```python
from build123d import *

# Parameters (mm, degrees)
SKIZZE1_W                            = 12
SKIZZE1_H                            = 17
AUFSATZ_LINEAR_AUSTRAGEN1_DEPTH      = 2
SCHNITT_LINEAR_AUSTRAGEN1_DEPTH      = 21.90454496
SCHNITT_LINEAR_AUSTRAGEN1_DEPTH_BACK = 21.90454496
SKIZZE4_W                            = 3
SKIZZE4_H                            = 1
SCHNITT_LINEAR_AUSTRAGEN3_DEPTH      = 1
VERRUNDUNG1_R                        = 0.5
VERRUNDUNG2_R                        = 1.5
VERRUNDUNG3_R                        = 0.25


# Some blends are built 0.0001 mm under size
with BuildPart() as part:
    # Skizze1 → Aufsatz-Linear austragen1 (new body)
    with BuildSketch(Plane(origin=(0, 0, 0), x_dir=(1, 0, 0), z_dir=(0, 1, 0))):
        with Locations((6, 8.5)):
            Rectangle(SKIZZE1_W, SKIZZE1_H)
    extrude(amount=AUFSATZ_LINEAR_AUSTRAGEN1_DEPTH)

    # Skizze4 → Schnitt-Linear austragen1 (cut, two sides: drawn at the far end of the back side and taken through both)
    with BuildSketch(Plane(origin=(0, 2, 0), x_dir=(1, 0, 0), z_dir=(0, 1, 0)).offset(-SCHNITT_LINEAR_AUSTRAGEN1_DEPTH_BACK)):
        with Locations((8.5, 2.5)):
            Rectangle(SKIZZE4_W, SKIZZE4_H)
        with Locations((3.5, 14.5)):
            Rectangle(SKIZZE4_W, SKIZZE4_H)
    extrude(amount=SCHNITT_LINEAR_AUSTRAGEN1_DEPTH + SCHNITT_LINEAR_AUSTRAGEN1_DEPTH_BACK, mode=Mode.SUBTRACT)

    # Skizze3 → Schnitt-Linear austragen3 (cut)
    with BuildSketch(Plane(origin=(0, 2, 0), x_dir=(1, 0, 0), z_dir=(0, 1, 0))):
        Polygon((8, 4), (3, 4), (3, 9), (8, 9), (8, 12), (3, 12), (3, 14), (2, 14), (2, 11), (7, 11), (7, 10), (2, 10), (2, 3), (8, 3), align=None)
        Polygon((9, 5), (4, 5), (4, 8), (9, 8), (9, 13), (4, 13), (4, 14), (10, 14), (10, 7), (5, 7), (5, 6), (10, 6), (10, 3), (9, 3), align=None)
    extrude(amount=-SCHNITT_LINEAR_AUSTRAGEN3_DEPTH, mode=Mode.SUBTRACT)

    # Verrundung1
    verrundung1_edges = [part.edges().sort_by_distance(p)[0] for p in [
        (3, 1.5, -12),
        (3, 1.5, -9),
        (7, 1.5, -3),
        (5, 1.5, -14),
        (9, 1.5, -5),
        (9, 1.5, -8),
        (9, 1.5, -13),
        (5, 1.5, -7),
        (5, 1.5, -6),
        (3, 1.5, -4),
        (7, 1.5, -10),
        (7, 1.5, -11),
    ]]
    fillet(verrundung1_edges, radius=VERRUNDUNG1_R - 0.0001)  # a hair under: the kernel refuses the full size

    # Verrundung2
    # the kernel refuses this fillet: 1.5 mm, written as the material it adds along each edge
    with BuildSketch(Plane(origin=(4, 2, -8), x_dir=(0, 0, 1), z_dir=(0, -1, 0)), Plane(origin=(2, 2, -11), x_dir=(1, 0, 0), z_dir=(0, -1, 0)), Plane(origin=(2, 2, -3), x_dir=(1, 0, 0), z_dir=(0, -1, 0)), Plane(origin=(2, 2, -10), x_dir=(0, 0, 1), z_dir=(0, -1, 0)), Plane(origin=(4, 2, -5), x_dir=(1, 0, 0), z_dir=(0, -1, 0))) as verrundung2_piece_1:
        with BuildLine():
            CenterArc((VERRUNDUNG2_R, -VERRUNDUNG2_R), VERRUNDUNG2_R, 90, 90)
            Line((0, -VERRUNDUNG2_R), (-VERRUNDUNG2_R * 0.02, -VERRUNDUNG2_R))
            Line((-VERRUNDUNG2_R * 0.02, -VERRUNDUNG2_R), (-VERRUNDUNG2_R * 0.02, VERRUNDUNG2_R * 0.02))
            Line((-VERRUNDUNG2_R * 0.02, VERRUNDUNG2_R * 0.02), (VERRUNDUNG2_R, VERRUNDUNG2_R * 0.02))
            Line((VERRUNDUNG2_R, VERRUNDUNG2_R * 0.02), (VERRUNDUNG2_R, 0))
        make_face()
    extrude(amount=1)
    with BuildSketch(Plane(origin=(8, 2, -4), x_dir=(-1, 0, 0), z_dir=(0, -1, 0)), Plane(origin=(4, 2, -13), x_dir=(1, 0, 0), z_dir=(0, -1, 0))) as verrundung2_piece_2:
        with BuildLine():
            CenterArc((1.414213562, -1.5), VERRUNDUNG2_R, 90, 70.528779366)
            Line((0, -1), (-0.028284271, -0.99))
            ThreePointArc((-0.028284271, -0.99), (-0.03, -0.5), (-0.03, 0))
            Line((-0.03, 0), (0, 0.03))
            Line((0, 0.03), (1.414213562, 0.03))
            Line((1.414213562, 0.03), (1.414213562, 0))
        make_face()
    extrude(amount=1)
    with BuildSketch(Plane(origin=(10, 2, -14), x_dir=(0, 0, 1), z_dir=(0, -1, 0)), Plane(origin=(10, 2, -7), x_dir=(-1, 0, 0), z_dir=(0, -1, 0)), Plane(origin=(10, 2, -6), x_dir=(0, 0, 1), z_dir=(0, -1, 0)), Plane(origin=(8, 2, -12), x_dir=(0, 0, 1), z_dir=(0, -1, 0)), Plane(origin=(8, 2, -9), x_dir=(-1, 0, 0), z_dir=(0, -1, 0))) as verrundung2_piece_3:
        with BuildLine():
            CenterArc((VERRUNDUNG2_R, VERRUNDUNG2_R), VERRUNDUNG2_R, 180, 90)
            Line((0, VERRUNDUNG2_R), (-VERRUNDUNG2_R * 0.02, VERRUNDUNG2_R))
            Line((-VERRUNDUNG2_R * 0.02, VERRUNDUNG2_R), (-VERRUNDUNG2_R * 0.02, -VERRUNDUNG2_R * 0.02))
            Line((-VERRUNDUNG2_R * 0.02, -VERRUNDUNG2_R * 0.02), (VERRUNDUNG2_R, -VERRUNDUNG2_R * 0.02))
            Line((VERRUNDUNG2_R, -VERRUNDUNG2_R * 0.02), (VERRUNDUNG2_R, 0))
        make_face()
    extrude(amount=1)

    # Verrundung3
    verrundung3_edges = [part.edges().sort_by_distance(p)[0] for p in [
        (3, 1.5, -14),
        (2.5, 1, -14),
        (5, 1, -14.24995),
        (7, 1, -2.75005),
        (10, 1, -2),
        (7, 1, -2),
        (2, 1, -15),
        (5, 1, -15),
        (4, 1.5, -14),
        (9, 1.5, -3),
        (4.5, 1, -14),
        (9.5, 1, -3),
        (7.5, 1, -3),
        (8, 1.5, -3),
    ]]
    fillet(verrundung3_edges, radius=VERRUNDUNG3_R)


solid = part.part
```
Check sheet for the modelled part. Datum: model origin and axes. Units: mm. A direction names the side the tool comes from. Give positions to 0.01 mm unless a question says otherwise; leave off trailing zeros. Write each loop counter-clockwise with the first axis right and the second up, starting at its lowest first coordinate (ties: lowest second). Pieces come first, ordered by that corner, then holes.
Item 1: Scan lines: L1, parallel to X at y = 1.45, z = -8.5; L2, parallel to Z at x = 3.5, y = 1.7; L3, parallel to X at y = 1.75, z = -10.25. Record each from-to range of solid material in increasing order.
Item 2: Cross-section at C-C (z = -9.25). Enter the section's corners in (x, y).
Item 3: Cross-section at B-B (x = 2.75). Enter the section's corners in (y, z), and give its area (3 significant figures).
Item 4: Cross-section at A-A (y = 0.3). Enter the section's corners in (x, z), and give its area (3 significant figures).
Item 5: Access from +Z, -Z, +X, -X, +Y, -Y to the whole of each face (thin tool, end or side, straight path). Record for faces 1 (the face through (8, 1, -2)), 2 (the face through (6, 2, -8.6)), 3 (the face through (2.45, 1.51, -3.43)).
Item 6: Draft check along Z on faces 4 (the face through (12, 1, -8)), 5 (the face through (2.45, 1.51, -11.43)), 6 (the face through (6, 1, 0)). Enter one of: released by +Z, released by -Z, zero draft, split by the parting line, or undercut.
Report:
1. L1: x = 0 to 2, 3 to 9, 10 to 12
1. L2: z = -17 to -15, -14 to -12, -11 to -10, -9 to -4, -3 to 0
1. L3: x = 0 to 6.93, 7.98 to 9, 10 to 12
2. outline: (0, 0) - (12, 0) - (12, 2) - (10, 2) - (10, 1) - (9, 1) - (9, 2) - (7.33, 2) - (7.33, 1) - (2.2, 1) - (2.2, 2) - (0, 2) - close
3. outline: (0, -17) - (2, -17) - (2, -15) - (0, -15) - close; (0, -14) - (0.75, -14) arc R0.25 ccw to (1, -13.75) - (1, -11.2) - (2, -11.2) - (2, -9.8) - (1, -9.8) - (1, -3.2) - (2, -3.2) - (2, 0) - (0, 0) - close
3. area: 22.6 mm2
4. outline: (0, -17) - (12, -17) - (12, 0) - (0, 0) - close; hole (2, -14.75) arc R0.25 ccw to (2.25, -15) - (4.75, -15) arc R0.25 ccw to (5, -14.75) - (5, -14) - (2, -14) - close; hole (7, -3) - (10, -3) - (10, -2.25) arc R0.25 ccw to (9.75, -2) - (7.25, -2) arc R0.25 ccw to (7, -2.25) - close
4. area: 198 mm2
5. face 1: +Y, -Y
5. face 2: +Z, -Z, +X, -X, +Y
5. face 3: +Y
6. face 4: zero draft
6. face 5: undercut
6. face 6: released by +Z
